Work out the finished part from the listing and answer in its coordinate system (mm). Face numbers are marked on the shaded views. Round coordinates to 2 decimals unless told otherwise and drop trailing zeros. Write each loop counter-clockwise with the first axis right and the second up, starting at its lowest first coordinate (ties: lowest second). Pieces come first, ordered by that corner, then holes. Notation, with made-up numbers: (36, 1) -> (40, 1) arc R31 ccw to (40, 39) -> close; hole circle Ø5 at (20, -21). An arc over 180 degrees is marked (long way). Answer as a JSON object with one key per item and string values. Group by question number.
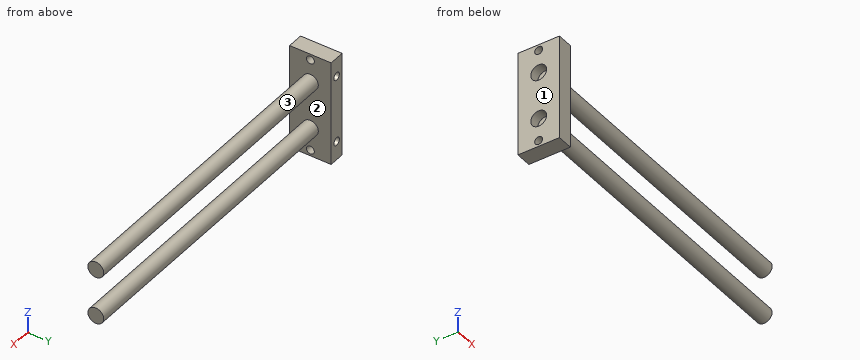
from build123d import *

# Parameters (mm, degrees)
SKETCH_1_W          = 53
SKETCH_1_H          = 21
SKETCH_1_R          = 2
EXTRUDE_1_DEPTH     = 8
SKETCH_2_R          = 4
CUT_EXTRUDE_1_DEPTH = 5
SKETCH_3_R          = 4
EXTRUDE_2_DEPTH     = 157
SKETCH_4_R          = 2
CUT_EXTRUDE_2_DEPTH = 5


with BuildPart() as part:
    # 草图1 → 凸台-拉伸1 (new body)
    with BuildSketch(Plane(origin=(0, 0, 0), x_dir=(0, 0, -1), z_dir=(1, 0, 0))):
        with Locations((26.5, 10.5)):
            Rectangle(SKETCH_1_W, SKETCH_1_H)
        with Locations((50, 10.5)):
            Circle(SKETCH_1_R, mode=Mode.SUBTRACT)
        with Locations(Location((3, 10.5, 0), (0, 0, 180))):
            Circle(SKETCH_1_R, mode=Mode.SUBTRACT)
    extrude(amount=EXTRUDE_1_DEPTH)

    # 草图2 → 切除-拉伸1 (cut)
    with BuildSketch(Plane.ZY):
        with Locations((-14.5, 10.5)):
            Circle(SKETCH_2_R)
        with Locations(Location((-38.5, 10.5, 0), (0, 0, 180))):
            Circle(SKETCH_2_R)
    extrude(amount=-CUT_EXTRUDE_1_DEPTH, mode=Mode.SUBTRACT)

    # 草图3 → 凸台-拉伸2 (add)
    with BuildSketch(Plane(origin=(8, 0, 0), x_dir=(0, 0, -1), z_dir=(1, 0, 0))):
        with Locations((38.5, 10.5)):
            Circle(SKETCH_3_R)
        with Locations(Location((14.5, 10.5, 0), (0, 0, 180))):
            Circle(SKETCH_3_R)
    extrude(amount=EXTRUDE_2_DEPTH)

    # 草图4 → 切除-拉伸2 (cut)
    with BuildSketch(Plane(origin=(0, 21, 0), x_dir=(1, 0, 0), z_dir=(0, 1, 0))):
        with Locations(Location((4, 43.5, 0), (0, 0, 270))):
            Circle(SKETCH_4_R)
        with Locations(Location((4, 9.5, 0), (0, 0, 90))):
            Circle(SKETCH_4_R)
    extrude(amount=-CUT_EXTRUDE_2_DEPTH, mode=Mode.SUBTRACT)


solid = part.part
1) A cutting plane is placed at D-D on x = 94. Determine the outline of the cut face in (y, z), plus the area to 3 significant figures.
2) A cutting plane is placed at A-A on z = -3. Determine the outline of the cut face in (x, y).
3) Straight lines are drawn through the part: L1, parallel to X at y = 19.55, z = -9.5; L2, parallel to Y at x = 3.05, z = -14.5; L3, parallel to Y at x = 2, z = -50. For each, find the intervals that lie inside material, in ascending order.
4) A cutting plane is placed at C-C on z = -14.5. Determine the outline of the cut face in (x, y).
5) For a pull along Z with two mould halves and no side action, classify the marked faces 1, 2 and 3 as released by +Z, released by -Z, zero draft, split by the parting line, or undercut.
6) A cutting plane is placed at B-B on y = 10.5. Determine the outline of the cut face in (x, z), plus the area to 3 significant figures.
7) Each of these flat-tipped pins is pushed along its axis until it touches: P1, Ø5, axis at x = 107, y = 9.5, coming from the -Z side; P2, Ø1, axis at x = 42, y = 9, coming from the +Z side; P3, Ø3.5, axis at y = 10.5, z = -3, coming from the -X side; P4, Ø10, axis at x = 32, z = -18.5, coming from the +Y side. Where does it stop, or does it pass through?
Established:
{
 "1": {"outline": "circle Ø8 at (10.5, -38.5); circle Ø8 at (10.5, -14.5)", "area": "101 mm²"},
 "2": {"outline": "(0, 0) -> (8, 0) -> (8, 8.5) -> (0, 8.5) -> close; (0, 12.5) -> (8, 12.5) -> (8, 21) -> (0, 21) -> close"},
 "3": {"L1": "x = 0 to 2, 6 to 8", "L2": "y = 0 to 6.5, 14.5 to 21", "L3": "y = 0 to 8.5, 12.5 to 21"},
 "4": {"outline": "(0, 0) -> (8, 0) -> (8, 6.5) -> (165, 6.5) -> (165, 14.5) -> (8, 14.5) -> (8, 21) -> (0, 21) -> (0, 14.5) -> (5, 14.5) -> (5, 6.5) -> (0, 6.5) -> close"},
 "5": {"face 1": "zero draft", "face 2": "undercut", "face 3": "undercut"},
 "6": {"outline": "(0, -53) -> (8, -53) -> (8, -52) -> (0, -52) -> close; (0, -48) -> (8, -48) -> (8, -42.5) -> (165, -42.5) -> (165, -34.5) -> (8, -34.5) -> (8, -18.5) -> (165, -18.5) -> (165, -10.5) -> (8, -10.5) -> (8, -5) -> (0, -5) -> (0, -10.5) -> (5, -10.5) -> (5, -18.5) -> (0, -18.5) -> (0, -34.5) -> (5, -34.5) -> (5, -42.5) -> (0, -42.5) -> close; (0, -1) -> (8, -1) -> (8, 0) -> (0, 0) -> close", "area": "2,790 mm²"},
 "7": {"P1": "stops at z = -42.5", "P2": "stops at z = -10.63", "P3": "passes through", "P4": "stops at y = 14.5"}
}
